```python
from build123d import *

# Parameters (mm, degrees)
BOSS_EXTRUDE4_DEPTH = 27.5
SKETCH2_W           = 19.5
SKETCH2_H           = 3
CUT_EXTRUDE1_DEPTH  = 240.335089361


with BuildPart() as part:
    # Sketch1 → Boss-Extrude4 (new, symmetric)
    with BuildSketch(Plane(origin=(0, 0, 0), x_dir=(1, 0, 0), z_dir=(0, 1, 0))):
        with BuildLine():
            Line((-185, 0), (185, 0))
            ThreePointArc((185, 0), (216.576404427, -12.938641896), (229.994773776, -44.314191845))
            Line((229.994773776, -44.314191845), (232.994425361, -44.268471301))
            ThreePointArc((232.994425361, -44.268471301), (218.681498055, -10.801218022), (185, 3))
            Line((185, 3), (-185, 3))
            ThreePointArc((-185, 3), (-218.681498055, -10.801218022), (-232.994425361, -44.268471301))
            Line((-232.994425361, -44.268471301), (-229.994773776, -44.314191845))
            ThreePointArc((-229.994773776, -44.314191845), (-216.576404427, -12.938641896), (-185, 0))
        make_face()
    extrude(amount=BOSS_EXTRUDE4_DEPTH, both=True)

    # Sketch2 → Cut-Extrude1 (cut, through all)
    with BuildSketch(Plane(origin=(0, 0, -3), x_dir=(-1, 0, 0), z_dir=(0, 0, -1))):
        with Locations((-125.25, -26)):
            Rectangle(SKETCH2_W, SKETCH2_H)
        with Locations((-175.25, -26)):
            Rectangle(SKETCH2_W, SKETCH2_H)
        with Locations((-75.25, -26)):
            Rectangle(SKETCH2_W, SKETCH2_H)
        with Locations((-25.25, -26)):
            Rectangle(SKETCH2_W, SKETCH2_H)
        with Locations((24.75, -26)):
            Rectangle(SKETCH2_W, SKETCH2_H)
        with Locations((74.75, -26)):
            Rectangle(SKETCH2_W, SKETCH2_H)
        with Locations((124.75, -26)):
            Rectangle(SKETCH2_W, SKETCH2_H)
        with Locations((174.75, -26)):
            Rectangle(SKETCH2_W, SKETCH2_H)
    extrude(amount=-CUT_EXTRUDE1_DEPTH, mode=Mode.SUBTRACT)


solid = part.part
```
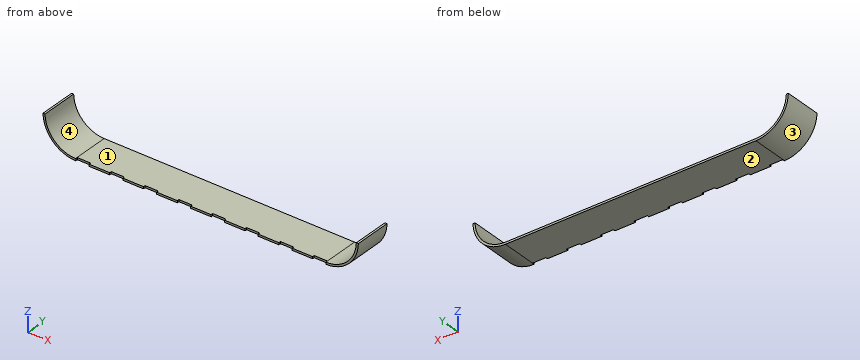
For this review, take the finished solid that the model builds, in its own axes (mm). Face numbers are marked on the shaded views. Give positions to 0.01 mm unless a question says otherwise; leave off trailing zeros. Write each loop counter-clockwise with the first axis right and the second up, starting at its lowest first coordinate (ties: lowest second). Pieces come first, ordered by that corner, then holes.
Item 1: Insertion check: P1, Ø10, axis at y = -20, z = 39, coming from the +X side; P2, Ø12, axis at y = -4.5, z = 5, coming from the +X side; P3, Ø6, axis at y = -0.5, z = 22, coming from the -X side. Each pin has a flat end and moves straight along its axis. Give the tip position at first contact, or say it passes through.
Item 2: Wall thickness on probe 1 along Z at (x, y) = (0, -21); probe 2 along X at (y, z) = (-9, 10); probe 3 along X at (y, z) = (4.5, 15): over which ranges is each line inside the solid? List them lowest first.
Item 3: Take a section at D-D (z = 31.5). Give the boundary of the cut face in (x, y).
Item 4: Take a section at A-A (z = 7). Give the boundary of the cut face in (x, y), and give its area (3 significant figures).
Item 5: The part is to be moulded in two halves that separate along X. For the marked faces 1, 2, 3 and 4, say which applies: +X half, -X half, draft (parallel to the pull), parting line (faces both ways), or undercut.
Item 6: Take a section at B-B (y = 2). Give the boundary of the cut face in (x, z).
Item 7: Take a section at C-C (x = 160.5). Give the boundary of the cut face in (y, z).
Established:
1. P1: stops at x = 232.99
1. P2: stops at x = 218.88
1. P3: stops at x = -228.63
2. probe 1: z = -3 to 0
2. probe 2: x = -217.85 to -213.28, 213.28 to 217.85
2. probe 3: x = -222.47 to -218.54, 218.54 to 222.47
3. outline: (-231.06, -27.5) - (-227.93, -27.5) - (-227.93, 27.5) - (-231.06, 27.5) - close; (227.93, -27.5) - (231.06, -27.5) - (231.06, 27.5) - (227.93, 27.5) - close
4. outline: (-214.33, -27.5) - (-209.1, -27.5) - (-209.1, 27.5) - (-214.33, 27.5) - close; (209.1, -27.5) - (214.33, -27.5) - (214.33, 27.5) - (209.1, 27.5) - close
4. area: 574 mm2
5. face 1: undercut
5. face 2: draft
5. face 3: -X half
5. face 4: undercut
6. outline: (-232.99, 44.27) arc R48 ccw to (-185, -3) - (185, -3) arc R48 ccw to (232.99, 44.27) - (229.99, 44.31) arc R45 cw to (185, 0) - (-185, 0) arc R45 cw to (-229.99, 44.31) - close
7. outline: (-27.5, -3) - (27.5, -3) - (27.5, 0) - (-27.5, 0) - close
